Source: CAD feature listing. Evaluate the final solid. Frame: model axes, mm. A direction names the side the tool comes from. Coordinates: 2 decimals unless noted, no trailing zeros. Order: outer loops, then holes, each group sorted by start corner. A loop starts at its lowest first (then second) coordinate and runs counter-clockwise, first axis right, second up. Notation, with made-up numbers: (24, -23) -> (77, -23) arc R20 cw to (77, 0) -> close; hole circle Ø2 at (67, 68.5). An arc over 180 degrees is marked (long way). Write each question's results on one line, items separated by ' | '. Start each with the question number.
from build123d import *

# Parameters (mm, degrees)
BOSS_EXTRUDE1_DEPTH = 5
BOSS_EXTRUDE2_DEPTH = 2
FILLET1_R           = 1


with BuildPart() as part:
    # Sketch1 → Boss-Extrude1 (new body)
    with BuildSketch(Plane(origin=(0, 0, 0), x_dir=(1, 0, 0), z_dir=(0, 1, 0))):
        Polygon((-4.5, -4.5), (-4.5, 58.5), (37.089540976, 58.5), (46.597851618, 47.242502808), (46.597851618, 12.6877701), (28.819604063, -4.5), align=None)
        Polygon((-0.5, -0.5), (-0.5, 54.5), (35.23217122, 54.5), (42.597851618, 45.779299812), (42.597851618, 14.384329511), (27.202178229, -0.5), align=None, mode=Mode.SUBTRACT)
    extrude(amount=BOSS_EXTRUDE1_DEPTH)

    # Sketch1_2 → Boss-Extrude2 (add)
    with BuildSketch(Plane(origin=(0, 0, 0), x_dir=(1, 0, 0), z_dir=(0, 1, 0))):
        Polygon((27.202178229, -0.5), (-0.5, -0.5), (-0.5, 54.5), (35.23217122, 54.5), (42.597851618, 45.779299812), (42.597851618, 14.384329511), align=None)
    extrude(amount=BOSS_EXTRUDE2_DEPTH)

    # Fillet1
    fillet1_edges = [part.edges().sort_by_distance(p)[0] for p in [
        (-4.5, 2.5, 4.5),
        (-4.5, 2.5, -58.5),
        (37.089540976, 2.5, -58.5),
        (46.597851618, 2.5, -47.242502808),
        (46.597851618, 2.5, -12.6877701),
        (28.819604063, 2.5, 4.5),
        (-0.5, 3.5, 0.5),
        (27.202178229, 3.5, 0.5),
        (42.597851618, 3.5, -14.384329511),
        (42.597851618, 3.5, -45.779299812),
        (35.23217122, 3.5, -54.5),
        (-0.5, 3.5, -54.5),
    ]]
    fillet(fillet1_edges, radius=FILLET1_R)


solid = part.part
(1) Section B-B on z = -42. Return the cut outline in (x, y).
(2) Draft query along X for faces 1 (the flat face through (21, 2, -27)), 2 (the flat face through (46.598, 2, -30)), 3 (the flat face through (16, 2, -58.5)). Return one class per face: released by +X, released by -X, zero draft, split by the parting line, or undercut.
(3) Line query: L1, parallel to X at y = 2.1, z = -22.5; L2, parallel to Z at x = 9.5, y = 4.7; L3, parallel to Y at x = 7, z = -21.5. Output: solid intervals per line, ascending.
(4) First-contact query: P1, Ø2, axis at x = 39.5, y = 4, coming from the +Z side. Flat tip, straight axial feed; report the tip coordinate or a pass-through.
(5) Section C-C on x = 13.5. Return the cut outline in (y, z).
(6) Reachability of faces 4 (the flat face through (14, 3, 0.5)), 5 (the flat face through (41.81, 2.46, -52.91)) from +Z, -Z, +X, -X, +Y, -Y: full face, straight path, thin tool, end or side. Return the list, or none.
(7) Section A-A on y = 3.2. Return the cut outline in (x, z).
Results list:
1) outline: (-4.5, 0) -> (46.6, 0) -> (46.6, 5) -> (42.6, 5) -> (42.6, 2) -> (-0.5, 2) -> (-0.5, 5) -> (-4.5, 5) -> close
2) face 1: undercut | face 2: released by +X | face 3: zero draft
3) L1: x = -4.5 to -0.5, 42.6 to 46.6 | L2: z = -58.5 to -54.5, 0.5 to 4.5 | L3: y = 0 to 2
4) P1: stops at z = -4.86
5) outline: (0, -58.5) -> (5, -58.5) -> (5, -54.5) -> (2, -54.5) -> (2, 0.5) -> (5, 0.5) -> (5, 4.5) -> (0, 4.5) -> close
6) face 4: +Y | face 5: -Z, +X, +Y, -Y
7) outline: (-4.5, -57.5) arc R1 ccw to (-3.5, -58.5) -> (36.63, -58.5) arc R1 ccw to (37.39, -58.15) -> (46.36, -47.52) arc R1 ccw to (46.6, -46.88) -> (46.6, -13.11) arc R1 ccw to (46.29, -12.39) -> (29.11, 4.22) arc R1 ccw to (28.42, 4.5) -> (-3.5, 4.5) arc R1 ccw to (-4.5, 3.5) -> close; hole (-0.5, -53.5) arc R1 ccw to (0.5, -54.5) -> (34.77, -54.5) arc R1 ccw to (35.53, -54.15) -> (42.36, -46.06) arc R1 ccw to (42.6, -45.41) -> (42.6, -14.81) arc R1 ccw to (42.29, -14.09) -> (27.49, 0.22) arc R1 ccw to (26.8, 0.5) -> (0.5, 0.5) arc R1 ccw to (-0.5, -0.5) -> close
